from build123d import *

# Parameters (mm, degrees)
F0_W            = 95
F0_H            = 65
F1_DEPTH        = 10
F2_W            = 93
F2_H            = 63
F3_DEPTH        = 8
F4_W            = 8
F4_H            = 30
F4_W_2          = 30
F4_H_2          = 8
F5_DEPTH        = 2
F6_T1_DEPTH     = 21.843134833
F6_T6_DEPTH     = 41.686269666
F6_T11_DEPTH    = 41.686269666
F7_C1_SIZE2     = 2
F7_C1_SIZE      = 5
F7_C2_SIZE2     = 5
F7_C2_SIZE      = 2
F7_C3_SIZE2     = 2
F7_C3_SIZE      = 5
F8_W            = 87
F8_H            = 8
F9_DEPTH        = 10
F10_SIZE        = 2.99999
F12_D           = 3.3
F12_CSINK_D     = 6.72
F12_CSINK_ANGLE = 90


# Not quite as in the source:
# - a fillet or chamfer that OpenCascade refuses, or shapes differently, is made with other operations: its cross-section is extruded or revolved along the edge and cut away or added
# - a fillet or chamfer is up to 0.001 mm smaller than in the source, because OpenCascade refuses the exact size


with BuildPart() as f1:
    # F0 (on Front) → F1 (new body)
    with BuildSketch(Plane.XZ):
        Rectangle(F0_W, F0_H)
    extrude(amount=F1_DEPTH)

    # F2 (on face) → F3 (cut)
    with BuildSketch(Plane.XZ.offset(10)):
        Rectangle(F2_W, F2_H)
    extrude(amount=-F3_DEPTH, mode=Mode.SUBTRACT)

    # F4 (on face) → F5 (join)
    with BuildSketch(Plane.XZ.offset(10)):
        with Locations((-43.5, 2.5)):
            Rectangle(F4_W, F4_H)
        with Locations((43.5, 2.5)):
            Rectangle(F4_W, F4_H)
        with Locations((2.5, -28.5)):
            Rectangle(F4_W_2, F4_H_2)
    extrude(amount=-F5_DEPTH)

    # F6: fillet of radius 8 on 6 edges, made by hand

    # F6_s2 → F6_t1 (cut)
    with BuildSketch(Plane.XZ.offset(8)):
        with BuildLine():
            ThreePointArc((-39.5, -4.5627460668), (-41.5, -9.8542486889), (-46.5, -12.5))
            Line((-46.5, -12.5), (-39.5, -12.5))
            Line((-39.5, -12.5), (-39.5, -4.5627460668))
        make_face()
        with BuildLine():
            ThreePointArc((-46.5, 17.5), (-41.5, 14.8542486889), (-39.5, 9.5627460668))
            Line((-39.5, 9.5627460668), (-39.5, 17.5))
            Line((-39.5, 17.5), (-46.5, 17.5))
        make_face()
        with BuildLine():
            ThreePointArc((-12.5, -31.5), (-9.8542486889, -26.5), (-4.5627460668, -24.5))
            Line((-4.5627460668, -24.5), (-12.5, -24.5))
            Line((-12.5, -24.5), (-12.5, -31.5))
        make_face()
        with BuildLine():
            ThreePointArc((9.5627460668, -24.5), (14.8542486889, -26.5), (17.5, -31.5))
            Line((17.5, -31.5), (17.5, -24.5))
            Line((17.5, -24.5), (9.5627460668, -24.5))
        make_face()
    extrude(amount=F6_T1_DEPTH, mode=Mode.SUBTRACT)


with BuildPart() as f6_tool4:
    # F6_s5 → F6_t6 (new body)
    with BuildSketch(Plane.XZ.offset(29.843134833)):
        with BuildLine():
            ThreePointArc((39.5, 9.5627460668), (41.5, 14.8542486889), (46.5, 17.5))
            Line((46.5, 17.5), (39.5, 17.5))
            Line((39.5, 17.5), (39.5, 9.5627460668))
        make_face()
    extrude(amount=-F6_T6_DEPTH)

    split(bisect_by=Plane.XZ.offset(2), keep=Keep.TOP)


with BuildPart() as f1_1:
    add(f1.part)

    # F6_t3: cut F6_tool4
    add(f6_tool4.part, mode=Mode.SUBTRACT)


with BuildPart() as f6_tool9:
    # F6_s10 → F6_t11 (new body)
    with BuildSketch(Plane.XZ.offset(29.843134833)):
        with BuildLine():
            ThreePointArc((46.5, -12.5), (41.5, -9.8542486889), (39.5, -4.5627460668))
            Line((39.5, -4.5627460668), (39.5, -12.5))
            Line((39.5, -12.5), (46.5, -12.5))
        make_face()
    extrude(amount=-F6_T11_DEPTH)

    split(bisect_by=Plane.XZ.offset(2), keep=Keep.TOP)


with BuildPart() as f1_2:
    add(f1_1.part)

    # F6_t8: cut F6_tool9
    add(f6_tool9.part, mode=Mode.SUBTRACT)

    # F7: chamfer of 2 x 5 on 3 edges, made by hand

    # F7_c1
    f7_c1_edges = [f1_2.edges().sort_by_distance(p)[0] for p in [
        (2.5, -8, -31.5),
    ]]
    f7_c1_side = f1_2.faces().sort_by_distance((2.5, -8, -31.46))[0]
    chamfer(f7_c1_edges, length=F7_C1_SIZE, length2=F7_C1_SIZE2, reference=f7_c1_side)

    # F7_c2
    f7_c2_edges = [f1_2.edges().sort_by_distance(p)[0] for p in [
        (-46.5, -8, 2.5),
    ]]
    f7_c2_side = f1_2.faces().sort_by_distance((-46.5, -7.96, 2.5))[0]
    chamfer(f7_c2_edges, length=F7_C2_SIZE, length2=F7_C2_SIZE2, reference=f7_c2_side)

    # F7_c3
    f7_c3_edges = [f1_2.edges().sort_by_distance(p)[0] for p in [
        (46.5, -8, 2.5),
    ]]
    f7_c3_side = f1_2.faces().sort_by_distance((46.5, -7.96, 2.5))[0]
    chamfer(f7_c3_edges, length=F7_C3_SIZE, length2=F7_C3_SIZE2, reference=f7_c3_side)

    # F8 (on face) → F9 (cut)
    with BuildSketch(Plane.XY.offset(32.5)):
        with Locations((0, -6)):
            Rectangle(F8_W, F8_H)
    extrude(amount=-F9_DEPTH, mode=Mode.SUBTRACT)

    # F10 (size 3 in the source; OpenCascade refuses exactly that, so slightly less here)
    f10_edges = [f1_2.edges().sort_by_distance(p)[0] for p in [
        (-46.5, -6, 31.5),
        (46.5, -6, 31.5),
    ]]
    chamfer(f10_edges, length=F10_SIZE)

    # F12 (through all)
    with Locations(Plane.XZ.offset(2)):
        with Locations((34.1857404726, 24.5), (-33.2815715389, 24.5)):
            CounterSinkHole(F12_D / 2, F12_CSINK_D / 2, counter_sink_angle=F12_CSINK_ANGLE)


solid = f1_2.part
CAD build for the part. Positions are in the model's coordinates, mm. A direction names the side the tool comes from. Coordinates: 2 decimals unless noted, no trailing zeros. Write each loop counter-clockwise with the first axis right and the second up, starting at its lowest first coordinate (ties: lowest second). Pieces come first, ordered by that corner, then holes. Notation, with made-up numbers: (71.5, 18.5) - (120.5, 18.5) arc R31 ccw to (120.5, 50.5) - close; hole circle Ø1 at (1, -16). An arc over 180 degrees is marked (long way). Use a Markdown table: item, result. Add a question column.
Item 1: Mould opens along Y. For faces 1 (the face through (-44, -7, 3)), 2 (the face through (32.5, -0.4, 25)), 3 (the face through (2, -9, -24.5)) say: pulls with the +Y half, pulls with the -Y half, needs draft (parallel to the pull), parting line crosses it, or undercut.
Item 2: Flat gauge pins, fed straight in: pin 1 (1 mm diameter, centred on x = -40.5, z = 1, fed in from +Y); pin 2 (4 mm diameter, centred on x = 33.5, z = -17, fed in from -Y); pin 3 (4.5 mm diameter, centred on x = -33.28, z = 24.5, fed in from -Y); pin 4 (2 mm diameter, centred on x = 2, y = -6, fed in from +Z). Where does each tip first touch, or does it go through?
Item 3: Band-saw the part on A-A, the plane z = 24.5. Give the cut face in (x, y), and give its area (3 significant figures).
Item 4: Drill centre lines: L1, parallel to X at y = -0.2, z = 24.5; L2, parallel to X at y = -7.5, z = -29.5; L3, parallel to X at y = -4, z = -24.5. Where is each one in solid material? Low to high. Write a range as from..to.
Item 5: Band-saw the part on D-D, the plane x = 1.5. Give the cut face in (y, z), and give its area (3 significant figures).
Item 6: 3-axis set-ups, long thin cutter, end or side, ignore diameter. For faces 4 (the face through (-41, -8, 3)), 5 (the face through (42.49, -8.88, -10.8)), 6 (the face through (15.694, -8.861, -27.361)), 7 (the face through (0, -1, 32.5)), 8 (the face through (42, -8, 3)): which of +Z, -Z, +X, -X, +Y, -Y reach the whole face in a straight line?
Item 7: Band-saw the part on C-C, the plane z = -16.5. Give the cut face in (x, y).
Numbers:
| question | item | result |
|---|---|---|
| 1 | face 1 | undercut |
| 1 | face 2 | pulls with the -Y half |
| 1 | face 3 | needs draft |
| 2 | pin 1 | y = 0 |
| 2 | pin 2 | y = -2 |
| 2 | pin 3 | y = -0.89 |
| 2 | pin 4 | z = -29 |
| 3 | outline | (-47.5, -10) - (-46.5, -10) - (-46.5, -2) - (-36.64, -2) - (-34.93, -0.29) - (-34.93, 0) - (-47.5, 0) - close; (-31.63, -0.29) - (-29.92, -2) - (30.83, -2) - (32.54, -0.29) - (32.54, 0) - (-31.63, 0) - close; (35.84, -0.29) - (37.55, -2) - (46.5, -2) - (46.5, -10) - (47.5, -10) - (47.5, 0) - (35.84, 0) - close |
| 3 | area | 187 mm2 |
| 4 | L1 | -47.5..-34.93, -31.63..32.54, 35.84..47.5 |
| 4 | L2 | -47.5..-46.5, -11.98..16.98, 46.5..47.5 |
| 4 | L3 | -47.5..-46.5, 46.5..47.5 |
| 5 | outline | (-10, -32.5) - (0, -32.5) - (0, 32.5) - (-2, 32.5) - (-2, -31.5) - (-6, -31.5) - (-8, -26.5) - (-8, -24.5) - (-10, -24.5) - close |
| 5 | area | 157 mm2 |
| 6 | face 4 | +Z |
| 6 | face 5 | -Y |
| 6 | face 6 | +Z, -Y |
| 6 | face 7 | +Z, +X, -X, +Y, -Y |
| 6 | face 8 | none |
| 7 | outline | (-47.5, -10) - (-46.5, -10) - (-46.5, -2) - (46.5, -2) - (46.5, -10) - (47.5, -10) - (47.5, 0) - (-47.5, 0) - close |
